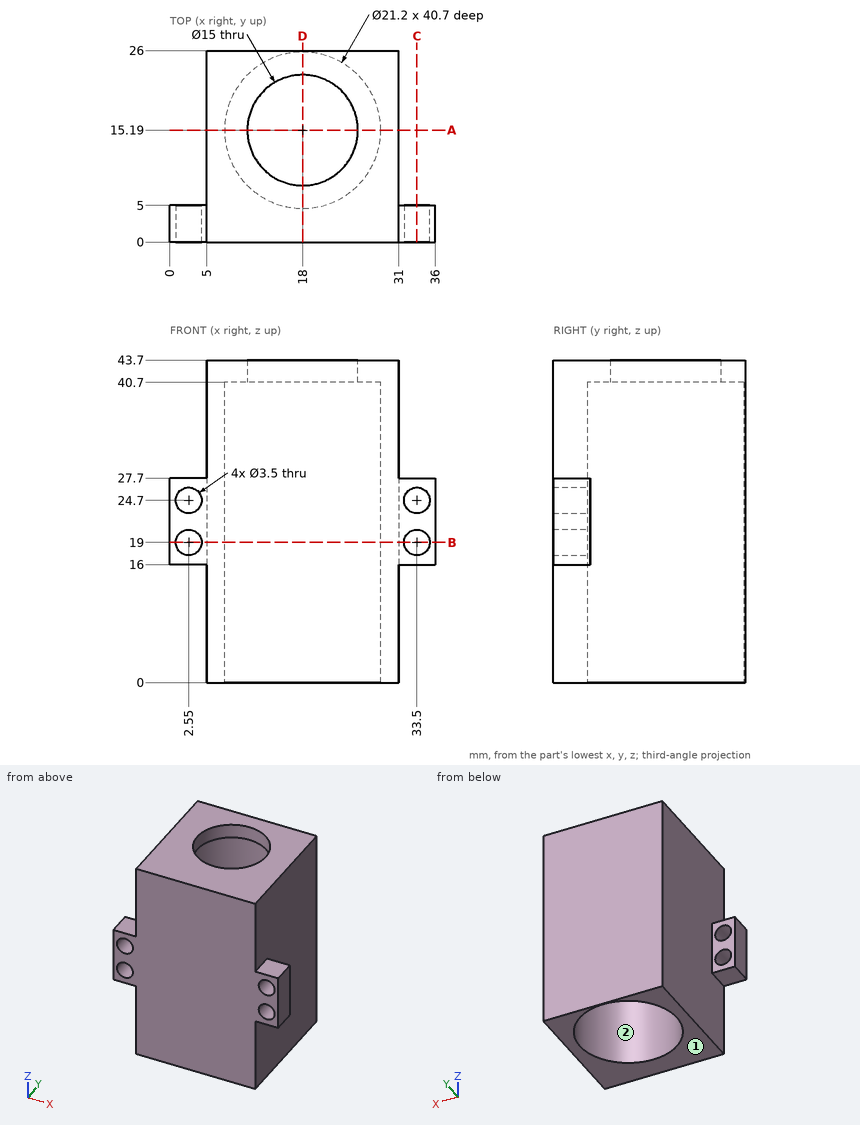
Design review of the part shown in the three views and the two pictorial views. Dimensions are in mm from the part's minimum x, y and z. Coordinates: 2 decimals unless noted, no trailing zeros. Write each loop counter-clockwise with the first axis right and the second up, starting at its lowest first coordinate (ties: lowest second). Pieces come first, ordered by that corner, then holes. Notation, with made-up numbers: (79.25, 84) - (121.25, 84) arc R17 ccw to (121.25, 113) - close; hole circle Ø1 at (40.25, 4.5). An arc over 180 degrees is marked (long way). Write item = value, one per line.
(1) Consider section B-B, the plane z = 19. Give the boundary of the cut face in (x, y), then the cut area to 3 significant figures.
Result sheet:
outline = (0, 0) - (0.8, 0) - (0.8, 5) - (0, 5) - close; (4.3, 0) - (31.75, 0) - (31.75, 5) - (31, 5) - (31, 26) - (5, 26) - (5, 5) - (4.3, 5) - close; (35.25, 0) - (36, 0) - (36, 5) - (35.25, 5) - close; hole circle Ø21.2 at (18, 15.19)
area = 338 mm^2
(2) Mouldability with a two-part tool opening along X and no side actions: class the marked faces 1 and 2 as pulls with the +X half, pulls with the -X half, needs draft (parallel to the pull), parting line crosses it, or undercut.
Result sheet:
face_1 = needs draft
face_2 = undercut
(3) Consider section A-A, the plane y = 15.19. Give the boundary of the cut face in (x, z).
Result sheet:
outline = (5, 0) - (7.4, 0) - (7.4, 40.7) - (10.5, 40.7) - (10.5, 43.7) - (5, 43.7) - close; (25.5, 40.7) - (28.6, 40.7) - (28.6, 0) - (31, 0) - (31, 43.7) - (25.5, 43.7) - close
(4) For P1, Ø2, axis at y = 9, z = 9, coming from the +X side; P2, Ø4, axis at x = 34, z = 21.5, coming from the +Y side; P3, Ø9, axis at x = 18, y = 15.19, coming from the +Z side; P4, Ø2.5, axis at x = 3, y = 2, coming from the +Z side, all flat-tipped, find the tip position at first contact; note any pin that passes through.
Result sheet:
P1 = 31
P2 = 5
P3 = through
P4 = 27.7
(5) Consider section C-C, the plane x = 33.5. Give the boundary of the cut face in (y, z).
Result sheet:
outline = (0, 16) - (5, 16) - (5, 17.25) - (0, 17.25) - close; (0, 20.75) - (5, 20.75) - (5, 22.95) - (0, 22.95) - close; (0, 26.45) - (5, 26.45) - (5, 27.7) - (0, 27.7) - close
(6) For line 1 (Z direction, x = 33.5, y = 3); line 2 (Y direction, x = 18, z = 16); line 3 (Z direction, x = 27, y = 15.25), list the stretches that pass through material, from the lowest coordinate up. Write a range as [from, to].
Result sheet:
line_1 = [16, 17.25], [20.75, 22.95], [26.45, 27.7]
line_2 = [0, 4.59], [25.79, 26]
line_3 = [40.7, 43.7]
(7) Consider section D-D, the plane x = 18. Give the boundary of the cut face in (y, z).
Result sheet:
outline = (0, 0) - (4.59, 0) - (4.59, 40.7) - (7.69, 40.7) - (7.69, 43.7) - (0, 43.7) - close; (22.69, 40.7) - (25.79, 40.7) - (25.79, 0) - (26, 0) - (26, 43.7) - (22.69, 43.7) - close
